```python
from build123d import *

# Parameters (mm, degrees)
SKETCH1_W           = 12.7
SKETCH1_H           = 31.75
SKETCH1_R           = 2.0828
BOSS_EXTRUDE1_DEPTH = 12.7
SKETCH2_R           = 2.0828
CUT_EXTRUDE1_DEPTH  = 12.7
SKETCH3_R           = 2.0828
CUT_EXTRUDE2_DEPTH  = 12.7


with BuildPart() as part:
    # Sketch1 → Boss-Extrude1 (new body)
    with BuildSketch(Plane(origin=(0, 0, 0), x_dir=(1, 0, 0), z_dir=(0, 1, 0))):
        with Locations((6.35, 15.875)):
            Rectangle(SKETCH1_W, SKETCH1_H)
        with Locations(Location((6.35, 18.034, 0), (0, 0, 270))):
            Circle(SKETCH1_R, mode=Mode.SUBTRACT)
    extrude(amount=BOSS_EXTRUDE1_DEPTH)

    # Sketch2 → Cut-Extrude1 (cut)
    with BuildSketch(Plane.XY):
        with Locations((6.35, 6.35)):
            Circle(SKETCH2_R)
    extrude(amount=-CUT_EXTRUDE1_DEPTH, mode=Mode.SUBTRACT)

    # Sketch3 → Cut-Extrude2 (cut)
    with BuildSketch(Plane.ZY):
        with Locations((-25.4, 6.35)):
            Circle(SKETCH3_R)
    extrude(amount=-CUT_EXTRUDE2_DEPTH, mode=Mode.SUBTRACT)


solid = part.part
```
Geometry check sheet. Reference: the model listing, model coordinates, mm. A direction names the side the tool comes from. Coordinates: 2 decimals unless noted, no trailing zeros. Write each loop counter-clockwise with the first axis right and the second up, starting at its lowest first coordinate (ties: lowest second). Pieces come first, ordered by that corner, then holes. Notation, with made-up numbers: M 27,21.5 L 59,21.5 A12 ccw 59,42.5 Z; hole C 0.25,50 d4. An arc over 180 degrees is marked long. One line per item, written item: value. Start each with the question number.
(1) Sectioned sample at C-C, the plane x = 6.35. Enter the section's corners in (y, z).
(2) Scan lines: line 1 along Y through (x, z) = (6.35, -9.25); line 2 along Z through (x, y) = (1.75, 6.5); line 3 along Z through (x, y) = (7.75, 7.5). Record each from-to range of solid material in increasing order. Write a range as [from, to].
(3) Sectioned sample at A-A, the plane y = 6.35. Enter the section's corners in (x, z).
(4) Release check for a two-part mould opening along X. For faces 3 (the face through (4.27, 6.44, -6.26)), 4 (the face through (6.26, 6.44, -27.48)), 5 (the face through (12.7, 6, -16)) record: released by +X, released by -X, zero draft, split by the parting line, or undercut.
(5) Sectioned sample at D-D, the plane y = 11.75. Enter the section's corners in (x, z).
(6) Tool access check on faces 1 (the face through (6, 6, -12.7)), 2 (the face through (6, 3, 0)). Record the directions out of +Z, -Z, +X, -X, +Y, -Y that give a thin tool (end or side, any length) a straight path to the whole face; none if there is none.
(7) Sectioned sample at B-B, the plane z = -25.4. Enter the section's corners in (x, y).
(8) Depth check by flat-ended pin: pin 1 (2 mm diameter, centred on x = 5.5, y = 7.5, fed in from +Z); pin 2 (3.5 mm diameter, centred on x = 6.35, z = -18.034, fed in from -Y); pin 3 (1.2 mm diameter, centred on x = 7, y = 7.5, fed in from +Z). Enter the tip coordinate at first touch or a pass-through.
Filled sheet:
1. outline: M 0,-31.75 L 12.7,-31.75 L 12.7,-20.12 L 0,-20.12 Z; M 0,-15.95 L 12.7,-15.95 L 12.7,0 L 8.43,0 L 8.43,-12.7 L 4.27,-12.7 L 4.27,0 L 0,0 Z; hole C 6.35,-25.4 d4.17
2. line 1: [0, 4.27], [8.43, 12.7]
2. line 2: [-31.75, -27.48], [-23.32, 0]
2. line 3: [-31.75, -27.14], [-23.66, -19.58], [-16.49, -12.7]
3. outline: M 0,-31.75 L 12.7,-31.75 L 12.7,-27.48 L 0,-27.48 Z; M 0,-23.32 L 12.7,-23.32 L 12.7,0 L 8.43,0 L 8.43,-12.7 L 4.27,-12.7 L 4.27,0 L 0,0 Z; hole C 6.35,-18.03 d4.17
4. face 3: undercut
4. face 4: zero draft
4. face 5: released by +X
5. outline: M 0,-31.75 L 12.7,-31.75 L 12.7,0 L 0,0 Z; hole C 6.35,-18.03 d4.17
6. face 1: +Z
6. face 2: +Z, +X, -X, +Y, -Y
7. outline: M 0,0 L 12.7,0 L 12.7,4.27 L 0,4.27 Z; M 0,8.43 L 12.7,8.43 L 12.7,12.7 L 0,12.7 Z
8. pin 1: z = 0
8. pin 2: through
8. pin 3: z = -12.7
